Design review of the part built by this model. Coordinates are the model's own, in mm. A direction names the side the tool comes from. Coordinates: 2 decimals unless noted, no trailing zeros. Loops run counter-clockwise (first coordinate to the right, second up) from the corner with the lowest first, then second, coordinate; pieces in that order, holes last. Notation, with made-up numbers: (28, 28.5) -> (32, 28.5) arc R27 ccw to (32, 44.5) -> close; hole circle Ø3 at (15, 54). An arc over 180 degrees is marked (long way). Answer in a Markdown table with one row per item.
```python
from build123d import *

# Parameters (mm, degrees)
SKETCH1_W           = 22
SKETCH1_H           = 3
BOSS_EXTRUDE1_DEPTH = 11.8
SKETCH1_3_W         = 22
SKETCH1_3_H         = 0.9
BOSS_EXTRUDE2_DEPTH = 5.6
CUT_EXTRUDE1_REACH  = 18.597
SKETCH2_R           = 1.1


with BuildPart() as part:
    # Sketch1 → Boss-Extrude1 (new body)
    with BuildSketch(Plane(origin=(0, 0, 0), x_dir=(1, 0, 0), z_dir=(0, 1, 0))):
        with Locations((0, 0.45)):
            Rectangle(SKETCH1_W, SKETCH1_H)
    extrude(amount=BOSS_EXTRUDE1_DEPTH)

    # Sketch1<3> → Boss-Extrude2 (add)
    with BuildSketch(Plane(origin=(0, 0, 0), x_dir=(1, 0, 0), z_dir=(0, 1, 0))):
        with Locations((0, -1.5)):
            Rectangle(SKETCH1_3_W, SKETCH1_3_H)
    extrude(amount=BOSS_EXTRUDE2_DEPTH)

    # Cut-Extrude1: up to this face of the body (flat: up to its plane)
    cut_extrude1_end = Plane(part.part.faces().sort_by_distance((0, 2.8, 1.95))[0])
    # Sketch2 → Cut-Extrude1 (cut, up to the picked face)
    with BuildSketch(Plane(origin=(0, 0, -1.95), x_dir=(-1, 0, 0), z_dir=(0, 0, -1)), mode=Mode.PRIVATE) as cut_extrude1_sk1:
        with Locations((-8.5, 2.8)):
            Circle(SKETCH2_R)
    cut_extrude1_tool1 = split(extrude(cut_extrude1_sk1.sketch, amount=-CUT_EXTRUDE1_REACH, mode=Mode.PRIVATE), bisect_by=cut_extrude1_end, keep=Keep.BOTH, mode=Mode.PRIVATE)
    # Sketch2 → Cut-Extrude1 (cut, up to the picked face)
    with BuildSketch(Plane(origin=(0, 0, -1.95), x_dir=(-1, 0, 0), z_dir=(0, 0, -1)), mode=Mode.PRIVATE) as cut_extrude1_sk2:
        with Locations((-8, 8.3)):
            Circle(SKETCH2_R)
    cut_extrude1_tool2 = split(extrude(cut_extrude1_sk2.sketch, amount=-CUT_EXTRUDE1_REACH, mode=Mode.PRIVATE), bisect_by=cut_extrude1_end, keep=Keep.BOTH, mode=Mode.PRIVATE)
    cut_extrude1_1 = cut_extrude1_tool1.solids().sort_by(Axis((8.5, 2.8, -1.95), (0, 0, 1)))[0]
    add(cut_extrude1_1, mode=Mode.SUBTRACT)
    cut_extrude1_2 = cut_extrude1_tool2.solids().sort_by(Axis((8, 8.3, -1.95), (0, 0, 1)))[0]
    add(cut_extrude1_2, mode=Mode.SUBTRACT)
    cut_extrude1 = cut_extrude1_1 + cut_extrude1_2  # Cut-Extrude1 as one shape, for the pattern or mirror that repeats it

    # Mirror1: Cut-Extrude1 across plane
    add(cut_extrude1.mirror(Plane(origin=(0, 0, 0), x_dir=(0, 0, 1), z_dir=(1, 0, 0))), mode=Mode.SUBTRACT)


solid = part.part
```
(1) For pin 1 (3.5 mm diameter, centred on x = 8.5, y = 2.8, fed in from +Z); pin 2 (2 mm diameter, centred on x = 2, y = 10.5, fed in from +Z); pin 3 (0.7 mm diameter, centred on x = -2, z = 1.5, fed in from +Y), all flat-tipped, find the tip position at first contact; note any pin that passes through.
Evaluation:
| item | result |
|---|---|
| pin 1 | stops at z = 1.95 |
| pin 2 | stops at z = 1.05 |
| pin 3 | stops at y = 5.6 |
(2) Take a section at B-B on z = -1. Give the boundary of the cut face in (x, y).
Evaluation:
| item | result |
|---|---|
| outline | (-11, 0) -> (11, 0) -> (11, 11.8) -> (-11, 11.8) -> close; hole circle Ø2.2 at (-8.5, 2.8); hole circle Ø2.2 at (-8, 8.3); hole circle Ø2.2 at (8, 8.3); hole circle Ø2.2 at (8.5, 2.8) |
(3) Draft analysis for pull direction X (two halves, no side actions). For faces 3 (the flat face through (-11, 6, 0)), 4 (the cylindrical face through (-7.484, 2.379, -0.027)), 5 (the flat face through (11, 6, 0)), 6 (the cylindrical face through (-7.41, 9.23, -0.47)), state which applies: pulls with the +X half, pulls with the -X half, needs draft (parallel to the pull), parting line crosses it, or undercut.
Evaluation:
| item | result |
|---|---|
| face 3 | pulls with the -X half |
| face 4 | undercut |
| face 5 | pulls with the +X half |
| face 6 | undercut |
(4) Take a section at D-D on z = 1.3. Give the boundary of the cut face in (x, y), and give its area (3 significant figures).
Evaluation:
| item | result |
|---|---|
| outline | (-11, 0) -> (11, 0) -> (11, 5.6) -> (-11, 5.6) -> close; hole circle Ø2.2 at (-8.5, 2.8); hole circle Ø2.2 at (8.5, 2.8) |
| area | 116 mm² |
(5) Take a section at A-A on y = 2.8. Give the boundary of the cut face in (x, z), and give its area (3 significant figures).
Evaluation:
| item | result |
|---|---|
| outline | (-11, -1.95) -> (-9.6, -1.95) -> (-9.6, 1.95) -> (-11, 1.95) -> close; (-7.4, -1.95) -> (7.4, -1.95) -> (7.4, 1.95) -> (-7.4, 1.95) -> close; (9.6, -1.95) -> (11, -1.95) -> (11, 1.95) -> (9.6, 1.95) -> close |
| area | 68.6 mm² |
(6) Take a section at C-C on x = 8. Give the boundary of the cut face in (y, z).
Evaluation:
| item | result |
|---|---|
| outline | (0, -1.95) -> (1.82, -1.95) -> (1.82, 1.95) -> (0, 1.95) -> close; (3.78, -1.95) -> (7.2, -1.95) -> (7.2, 1.05) -> (5.6, 1.05) -> (5.6, 1.95) -> (3.78, 1.95) -> close; (9.4, -1.95) -> (11.8, -1.95) -> (11.8, 1.05) -> (9.4, 1.05) -> close |
(7) To check wall thickness, follow probe 1 along X at (y, z) = (2, 0.1); probe 2 along X at (y, z) = (7.75, -0.3); probe 3 along Y at (x, z) = (8, 0.25). State the ranges of each line that lie inside material, in increasing order.
Evaluation:
| item | result |
|---|---|
| probe 1 | x = -11 to -9.25, -7.75 to 7.75, 9.25 to 11 |
| probe 2 | x = -11 to -8.95, -7.05 to 7.05, 8.95 to 11 |
| probe 3 | y = 0 to 1.82, 3.78 to 7.2, 9.4 to 11.8 |
(8) Tool access review of faces 1 (the cylindrical face through (7.484, 2.379, -0.027)), 2 (the flat face through (-0.2, 5.6, 1.5)): name each direction out of +Z, -Z, +X, -X, +Y, -Y from which nothing blocks a thin tool from reaching the whole face with its end or side.
Evaluation:
| item | result |
|---|---|
| face 1 | +Z, -Z |
| face 2 | +Z, +X, -X, +Y |
